For this review, use the dimensioned drawing (mm, ordinates from the lowest corner) and the shaded views. A direction names the side the tool comes from. Give positions to 0.01 mm unless a question says otherwise; leave off trailing zeros. Loops run counter-clockwise (first coordinate to the right, second up) from the corner with the lowest first, then second, coordinate; pieces in that order, holes last. Notation, with made-up numbers: (-32, 84) - (-23, 84) arc R20 cw to (-23, 109) - close; hole circle Ø2 at (32.5, -27.5). An arc over 180 degrees is marked (long way). Put each result on its own line as item: value.
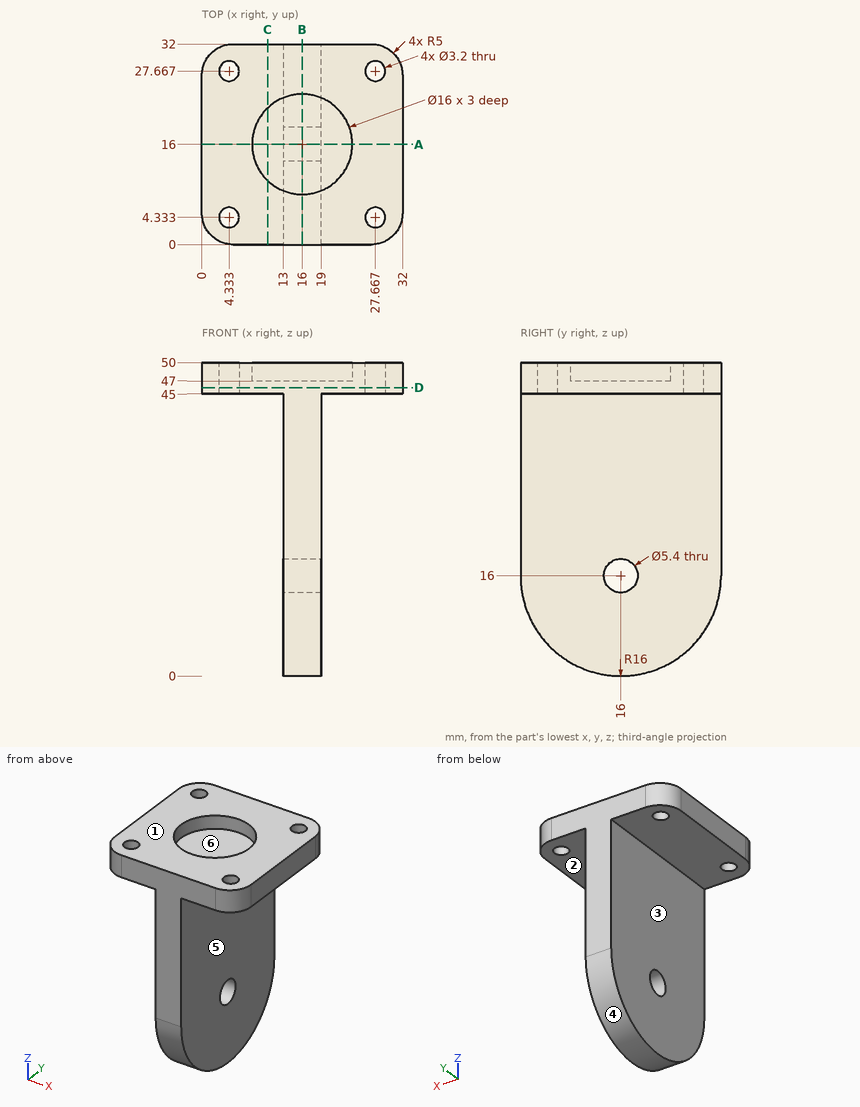
1) Take a section at D-D on z = 46. State the section outline as (x, y) points, and give its area (3 significant figures).
Geometry check:
outline: (0, 5) arc R5 ccw to (5, 0) - (27, 0) arc R5 ccw to (32, 5) - (32, 27) arc R5 ccw to (27, 32) - (5, 32) arc R5 ccw to (0, 27) - close; hole circle Ø3.2 at (4.33, 4.33); hole circle Ø3.2 at (4.33, 27.67); hole circle Ø3.2 at (27.67, 4.33); hole circle Ø3.2 at (27.67, 27.67)
area: 970 mm²
2) Wall thickness on line 1 (Y direction, x = 17.75, z = 16); line 2 (X direction, y = 19.5, z = 43.5); line 3 (Z direction, x = 12, y = 5.5): over which ranges is each line inside the solid? List them lowest first.
Geometry check:
line 1: y = 0 to 13.3, 18.7 to 32
line 2: x = 13 to 19
line 3: z = 45 to 50
3) Take a section at A-A on y = 16. State the section outline as (x, z) points.
Geometry check:
outline: (0, 45) - (13, 45) - (13, 18.7) - (19, 18.7) - (19, 45) - (32, 45) - (32, 50) - (24, 50) - (24, 47) - (8, 47) - (8, 50) - (0, 50) - close; (13, 0) - (19, 0) - (19, 13.3) - (13, 13.3) - close
4) Take a section at B-B on x = 16. State the section outline as (y, z) points, and give its area (3 significant figures).
Geometry check:
outline: (0, 16) arc R16 ccw to (32, 16) - (32, 50) - (24, 50) - (24, 47) - (8, 47) - (8, 50) - (0, 50) - close; hole circle Ø5.4 at (16, 16)
area: 1,420 mm²
5) Insertion check: pin 1 Ø8 at (y, z) = (14, 9.5) entering from +X; pin 2 Ø12 at (x, z) = (24.5, 10.5) entering from -Y; pin 3 Ø6 at (x, y) = (21.5, 21) entering from -Z; pin 4 Ø1.9 at (x, y) = (27.67, 27.67) entering from +Z (3 decimals). Each pin has a flat end and moves straight along its axis. Give the tip position at first contact, or say it passes through.
Geometry check:
pin 1: stops at x = 19
pin 2: stops at y = 0.3
pin 3: stops at z = 0.35
pin 4: passes through
6) Draft analysis for pull direction X (two halves, no side actions). For the marked faces 4, 5 and 6, state which applies: pulls with the +X half, pulls with the -X half, needs draft (parallel to the pull), parting line crosses it, or undercut.
Geometry check:
face 4: needs draft
face 5: pulls with the +X half
face 6: undercut
7) Take a section at C-C on x = 10.5. State the section outline as (y, z) points.
Geometry check:
outline: (0, 45) - (32, 45) - (32, 50) - (21.81, 50) - (21.81, 47) - (10.19, 47) - (10.19, 50) - (0, 50) - close
8) For the marked faces 1, 2 and 3, list the 3-axis set-ups (+Z, -Z, +X, -X, +Y, -Y) from which the entire face can be reached by the end or side of a thin tool; tool diameter is ignored.
Geometry check:
face 1: +Z, +X, -X, +Y, -Y
face 2: -Z, +X, +Y, -Y
face 3: -Z, -X, +Y, -Y
